Input: part model. Units: mm. Frame: model coordinates. A direction names the side the tool comes from. Give positions to 0.01 mm unless a question says otherwise; leave off trailing zeros. Loops run counter-clockwise (first coordinate to the right, second up) from the corner with the lowest first, then second, coordinate; pieces in that order, holes last. Notation, with made-up numbers: (39.5, 74.25) -> (75.5, 74.25) arc R28 cw to (75.5, 95.25) -> close; hole circle Ø7 at (0.25, -18.5). An arc over 180 degrees is marked (long way). Use CSV: the item, a comma, the result in double quotes.
```python
from build123d import *

# Parameters (mm, degrees)
BOSS_EXTRUDE1_DEPTH = 5
SKETCH2_W           = 5
SKETCH2_H           = 25
CUT_EXTRUDE1_DEPTH  = 164.135403883
FILLET1_R           = 10
SKETCH3_W           = 25
SKETCH3_H           = 5
CUT_EXTRUDE2_DEPTH  = 10
SKETCH4_W           = 60
SKETCH4_H           = 30
CUT_EXTRUDE3_DEPTH  = 35
FILLET2_R           = 10


with BuildPart() as part:
    # Sketch1 → Boss-Extrude1 (new body)
    with BuildSketch(Plane.XY):
        with BuildLine():
            Line((60, -105.6), (120, -105.6))
            Line((120, -105.6), (120, 70.4))
            Line((120, 70.4), (80, 70.4))
            ThreePointArc((80, 70.4), (72.928932188, 73.328932188), (70, 80.4))
            Line((70, 80.4), (70, 110.4))
            Line((70, 110.4), (-70, 110.4))
            Line((-70, 110.4), (-70, 80.4))
            ThreePointArc((-70, 80.4), (-72.928932188, 73.328932188), (-80, 70.4))
            Line((-80, 70.4), (-120, 70.4))
            Line((-120, 70.4), (-120, -105.6))
            Line((-120, -105.6), (-60, -105.6))
            Line((-60, -105.6), (-60, -100.6))
            ThreePointArc((-60, -100.6), (-58.535533906, -97.064466094), (-55, -95.6))
            Line((-55, -95.6), (55, -95.6))
            ThreePointArc((55, -95.6), (58.535533906, -97.064466094), (60, -100.6))
            Line((60, -100.6), (60, -105.6))
        make_face()
    extrude(amount=BOSS_EXTRUDE1_DEPTH)

    # Sketch2 → Cut-Extrude1 (cut, through all)
    with BuildSketch(Plane.XY.offset(5)):
        with Locations((102.75, 32.41)):
            Rectangle(SKETCH2_W, SKETCH2_H)
        with Locations((102.75, -8.59)):
            Rectangle(SKETCH2_W, SKETCH2_H)
        with Locations((102.75, -49.59)):
            Rectangle(SKETCH2_W, SKETCH2_H)
        with Locations((-101.25, 32.41)):
            Rectangle(SKETCH2_W, SKETCH2_H)
        with Locations((-101.25, -8.59)):
            Rectangle(SKETCH2_W, SKETCH2_H)
        with Locations((-101.25, -49.59)):
            Rectangle(SKETCH2_W, SKETCH2_H)
    extrude(amount=-CUT_EXTRUDE1_DEPTH, mode=Mode.SUBTRACT)

    # Fillet1
    fillet1_edges = [part.edges().sort_by_distance(p)[0] for p in [
        (-70, 110.4, 2.5),
        (70, 110.4, 2.5),
    ]]
    fillet(fillet1_edges, radius=FILLET1_R)

    # Sketch3 → Cut-Extrude2 (cut)
    with BuildSketch(Plane.XY.offset(5)):
        with Locations((62.25, -77.6)):
            Rectangle(SKETCH3_W, SKETCH3_H)
        with Locations((21.25, -77.6)):
            Rectangle(SKETCH3_W, SKETCH3_H)
        with Locations((-19.75, -77.6)):
            Rectangle(SKETCH3_W, SKETCH3_H)
        with Locations((-60.75, -77.6)):
            Rectangle(SKETCH3_W, SKETCH3_H)
    extrude(amount=-CUT_EXTRUDE2_DEPTH, mode=Mode.SUBTRACT)

    # Sketch4 → Cut-Extrude3 (cut)
    with BuildSketch(Plane.XY.offset(5)):
        with Locations((0, 80.204694575)):
            Rectangle(SKETCH4_W, SKETCH4_H)
    extrude(amount=-CUT_EXTRUDE3_DEPTH, mode=Mode.SUBTRACT)

    # Fillet2
    fillet2_edges = [part.edges().sort_by_distance(p)[0] for p in [
        (-30, 65.204694575, 2.5),
        (-30, 95.204694575, 2.5),
        (30, 95.204694575, 2.5),
        (30, 65.204694575, 2.5),
    ]]
    fillet(fillet2_edges, radius=FILLET2_R)


solid = part.part
```
1) Contact query for flat-ended pins moving along their axis: pin 1 (3 mm diameter, centred on x = 22, z = 1.5, fed in from -Y); pin 2 (1.5 mm diameter, centred on y = 89.5, z = 1.5, fed in from -X); pin 3 (2 mm diameter, centred on x = 62, y = 71, fed in from -Z). Output: stop coordinate, or through.
From the geometry:
pin 1,"stops at y = -95.6"
pin 2,"stops at x = -70"
pin 3,"stops at z = 0"
2) Ray query, line 1 (X direction, y = -42, z = 4.3); line 2 (Y direction, x = -19, z = 3.8); line 3 (X direction, y = 84, z = 3.85). Return the intervals inside material, ascending.
From the geometry:
line 1,"x = -120 to -103.75, -98.75 to 100.25, 105.25 to 120"
line 2,"y = -95.6 to -80.1, -75.1 to 65.2, 95.2 to 110.4"
line 3,"x = -70 to -30, 30 to 70"
3) Section query C-C (z = 4.05). Give the number of separate pieces and of enclosed holes in the cut face, then the cut area to 3 significant figures.
From the geometry:
separate pieces,"1"
enclosed holes,"11"
area,"43,700 mm^2"
4) Section query A-A (y = -12). Return loops of the section in (x, z), then the cut area to 3 significant figures.
From the geometry:
outline,"(-120, 0) -> (-103.75, 0) -> (-103.75, 5) -> (-120, 5) -> close; (-98.75, 0) -> (100.25, 0) -> (100.25, 5) -> (-98.75, 5) -> close; (105.25, 0) -> (120, 0) -> (120, 5) -> (105.25, 5) -> close"
area,"1,150 mm^2"
5) Reachability of faces 4 (the flat face through (49.75, -78, 3)), 5 (the flat face through (-60, -103, 2)), 6 (the flat face through (1, 110.4, 2)) from +Z, -Z, +X, -X, +Y, -Y: full face, straight path, thin tool, end or side. Return the list, or none.
From the geometry:
face 4,"+Z, -Z"
face 5,"+Z, -Z, -Y"
face 6,"+Z, -Z, +X, -X, +Y"
6) Section query B-B (x = -13.5). Return loops of the section in (y, z).
From the geometry:
outline,"(-95.6, 0) -> (-80.1, 0) -> (-80.1, 5) -> (-95.6, 5) -> close; (-75.1, 0) -> (65.2, 0) -> (65.2, 5) -> (-75.1, 5) -> close; (95.2, 0) -> (110.4, 0) -> (110.4, 5) -> (95.2, 5) -> close"
7) Section query D-D (x = 93). Return loops of the section in (y, z), then the cut area to 3 significant figures.
From the geometry:
outline,"(-105.6, 0) -> (70.4, 0) -> (70.4, 5) -> (-105.6, 5) -> close"
area,"880 mm^2"
8) Mould query, pull axis X, two halves, no side actions, for faces 1 (the flat face through (-2, -20, 0)), 2 (the flat face through (-120, -16, 2)), 3 (the flat face through (100.25, 32, 3)). Classes: pulls with the +X half, pulls with the -X half, needs draft (parallel to the pull), parting line crosses it, or undercut.
From the geometry:
face 1,"needs draft"
face 2,"pulls with the -X half"
face 3,"undercut"
